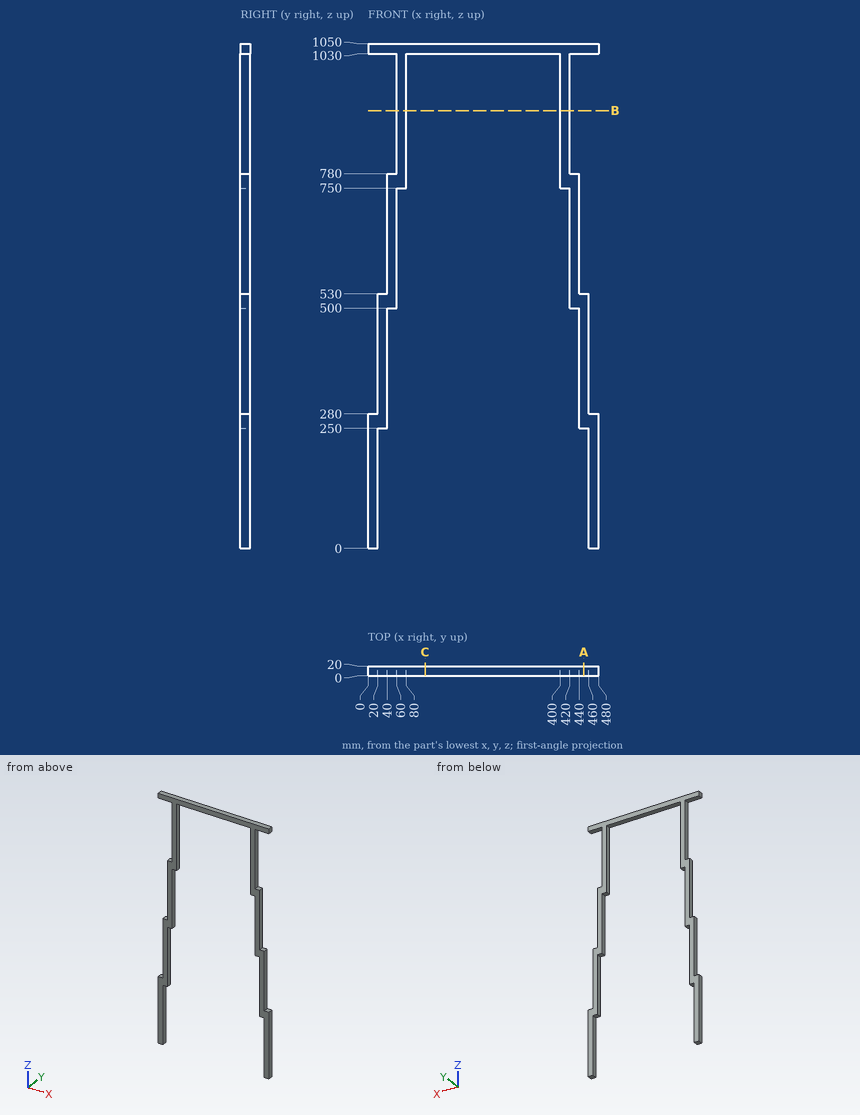
Can you work these out from the drawing? Everything is in mm from the part's minimum corner. Round coordinates to 2 decimals unless told otherwise and drop trailing zeros. Order: outer loops, then holes, each group sorted by start corner. A loop starts at its lowest first (then second) coordinate and runs counter-clockwise, first axis right, second up. Notation, with made-up numbers: M 55,-38.5 L 78,-38.5 A16 cw 78,-27.5 Z; hole C 49,45.25 d3. An arc over 180 degrees is marked long. One line per question, with ' | ' between items.
1) I want a section at B-B, the plane z = 911.5. Write out the boundary of the cut face in (x, y).
Working result:
outline: M 60,0 L 80,0 L 80,20 L 60,20 Z; M 400,0 L 420,0 L 420,20 L 400,20 Z
2) I want a section at C-C, the plane x = 119. Write out the boundary of the cut face in (y, z), then the cut area to 3 significant figures.
Working result:
outline: M 0,1030 L 20,1030 L 20,1050 L 0,1050 Z | area: 400 mm²
3) I need wall thicknesses on line 1 along X through (y, z) = (1.75, 266); line 2 along X through (y, z) = (9.25, 196); line 3 along Z through (x, y) = (427, 13.75). Which ranges of each line are inside material? Lowest first, please.
Working result:
line 1: 0 to 40, 440 to 480 | line 2: 0 to 20, 460 to 480 | line 3: 500 to 780, 1030 to 1050
4) I want a section at A-A, the plane x = 449.5. Write out the boundary of the cut face in (y, z).
Working result:
outline: M 0,250 L 20,250 L 20,530 L 0,530 Z; M 0,1030 L 20,1030 L 20,1050 L 0,1050 Z
5) For pin 1 Ø6 at (y, z) = (15, 600) entering from +X; pin 2 Ø2 at (y, z) = (14, 478.5) entering from -X; pin 3 Ø6 at (x, y) = (454.5, 10) entering from -Z, each with a flat end and sliding along its axis, tell me the tip position at first contact or that it passes through.
Working result:
pin 1: x = 440 | pin 2: x = 20 | pin 3: z = 250
